Verification items for the finished model (mm, model axes). A direction names the side the tool comes from. Give positions to 0.01 mm unless a question says otherwise; leave off trailing zeros. Loops run counter-clockwise (first coordinate to the right, second up) from the corner with the lowest first, then second, coordinate; pieces in that order, holes last. Notation, with made-up numbers: M -36,15 L 9,15 A23 ccw 9,29 Z; hole C -7.5,7 d7. An arc over 180 degrees is marked long. Use CSV: the item, a comma, the result in double quotes.
from build123d import *

# Parameters (mm, degrees)
SKETCH1_R                   = 20.701
BOSS_EXTRUDE1_DEPTH         = 25.4
SKETCH2_W                   = 25.654
SKETCH2_H                   = 101.6
CUT_EXTRUDE1_DEPTH          = 25.654
F_1_4_20_TAPPED_HOLE1_D     = 5.1054
F_1_4_20_TAPPED_HOLE1_DEPTH = 25.4
F_1_4_20_TAPPED_HOLE1_TIP   = 1.533816902
F_3_8_24_TAPPED_HOLE1_D     = 8.4328
SKETCH10_R                  = 9.525
CUT_EXTRUDE2_DEPTH          = 19.05
CHAMFER1_SIZE               = 1.27


with BuildPart() as part:
    # Sketch1 → Boss-Extrude1 (new, symmetric)
    with BuildSketch(Plane.XY):
        with BuildLine():
            Line((0, 0), (0, 203.2))
            ThreePointArc((0, 203.2), (44.636926547, 310.963073453), (152.4, 355.6))
            Line((152.4, 355.6), (285.75, 355.6))
            Line((285.75, 355.6), (285.75, 254))
            Line((285.75, 254), (203.2, 254))
            ThreePointArc((203.2, 254), (131.357951031, 224.242048969), (101.6, 152.4))
            Line((101.6, 152.4), (101.6, 0))
            Line((101.6, 0), (0, 0))
        make_face()
        with Locations((242.9256, 304.8)):
            Circle(SKETCH1_R, mode=Mode.SUBTRACT)
    extrude(amount=BOSS_EXTRUDE1_DEPTH, both=True)

    # Sketch2 → Cut-Extrude1 (cut)
    with BuildSketch(Plane(origin=(285.75, 0, 0), x_dir=(0, 0, -1), z_dir=(1, 0, 0))):
        with Locations((0, 304.8)):
            Rectangle(SKETCH2_W, SKETCH2_H)
    extrude(amount=-CUT_EXTRUDE1_DEPTH, mode=Mode.SUBTRACT)

    # 1/4-20 Tapped Hole1
    with Locations(Plane(origin=(285.75, 0, 0), x_dir=(0, 0, -1), z_dir=(1, 0, 0))):
        with Locations((19.05, 342.9), (-19.05, 342.9), (-19.05, 266.7), (19.05, 266.7)):
            Hole(F_1_4_20_TAPPED_HOLE1_D / 2, depth=F_1_4_20_TAPPED_HOLE1_DEPTH)
            with Locations((0, 0, -(F_1_4_20_TAPPED_HOLE1_DEPTH + F_1_4_20_TAPPED_HOLE1_TIP / 2))):  # 118° drill point
                Cone(0, F_1_4_20_TAPPED_HOLE1_D / 2, F_1_4_20_TAPPED_HOLE1_TIP, mode=Mode.SUBTRACT)

    # 3/8-24 Tapped Hole1 (through all)
    with Locations(Plane.XY.offset(25.4)):
        with Locations((12.7, 29.21), (12.7, 8.89)):
            Hole(F_3_8_24_TAPPED_HOLE1_D / 2)

    # Sketch10 → Cut-Extrude2 (cut)
    with BuildSketch(Plane(origin=(101.6, 0, 0), x_dir=(0, 0, -1), z_dir=(1, 0, 0))):
        with Locations(Location((0, 19.05, 0), (0, 0, 90))):
            Circle(SKETCH10_R)
    extrude(amount=-CUT_EXTRUDE2_DEPTH, mode=Mode.SUBTRACT)

    # Chamfer1
    chamfer1_edges = [part.edges().sort_by_distance(p)[0] for p in [
        (244.475, 254, -25.4),
        (131.357951031, 224.242048969, -25.4),
        (101.6, 76.2, -25.4),
        (131.357951031, 224.242048969, 25.4),
        (244.475, 254, 25.4),
        (219.075, 355.6, 25.4),
        (44.636926547, 310.963073453, 25.4),
        (0, 101.6, 25.4),
        (0, 101.6, -25.4),
        (101.6, 76.2, 25.4),
        (44.636926547, 310.963073453, -25.4),
        (219.075, 355.6, -25.4),
    ]]
    chamfer(chamfer1_edges, length=CHAMFER1_SIZE)


solid = part.part
(1) Section check A-A on y = 104.5. Record the cut outline in (x, z), plus the area to 3 significant figures.
Calculated:
outline,"M 0,-24.13 L 1.27,-25.4 L 100.33,-25.4 L 101.6,-24.13 L 101.6,24.13 L 100.33,25.4 L 1.27,25.4 L 0,24.13 Z"
area,"5,160 mm²"
(2) Mould release check, pull along Y, two halves, no side actions. Record for faces 4 (the flat face through (236, 254, 0)), 5 (the conical face through (44.2, 309, 25.2)), 6 (the cylindrical face through (13.25, 33.39, -0.36)), 7 (the flat face through (101.6, 77, 0)): released by +Y, released by -Y, zero draft, split by the parting line, or undercut.
Calculated:
face 4,"released by -Y"
face 5,"released by +Y"
face 6,"undercut"
face 7,"zero draft"
(3) Tool access check on faces 1 (the cylindrical face through (92.208, 11.491, -5.796)), 2 (the flat face through (260.096, 336, 0)), 3 (the flat face through (285.75, 306, 19)). Record the directions out of +Z, -Z, +X, -X, +Y, -Y that give a thin tool (end or side, any length) a straight path to the whole face; none if there is none.
Calculated:
face 1,"+X"
face 2,"+X, +Y, -Y"
face 3,"+Z, -Z, +X, +Y, -Y"
(4) Section check B-B on y = 19.05. Record the cut outline in (x, z) (3 decimals).
Calculated:
outline,"M 0,-24.13 L 1.27,-25.4 L 100.33,-25.4 L 101.6,-24.13 L 101.6,-9.525 L 82.55,-9.525 L 82.55,9.525 L 101.6,9.525 L 101.6,24.13 L 100.33,25.4 L 1.27,25.4 L 0,24.13 Z"
(5) Scan lines: L1, parallel to Y at x = 272, z = -19; L2, parallel to Z at x = 278, y = 266.7; L3, parallel to Y at x = 241.5, z = -16. Record each from-to range of solid material in increasing order. Write a range as from..to.
Calculated:
L1,"y = 254..264.15, 269.25..340.35, 345.45..355.6"
L2,"z = -25.4..-21.6, -16.5..-12.83, 12.83..16.5, 21.6..25.4"
L3,"y = 254..284.15, 325.45..355.6"
(6) Depth check by flat-ended pin: pin 1 Ø20.5 at (y, z) = (338, 1.5) entering from +X; pin 2 Ø8 at (y, z) = (285, 2.5) entering from -X; pin 3 Ø4.5 at (y, z) = (342.9, 19.05) entering from -X; pin 4 Ø8 at (y, z) = (342.9, -19.05) entering from +X. Enter the tip coordinate at first touch or a pass-through.
Calculated:
pin 1,"stops at x = 260.1"
pin 2,"stops at x = 21.35"
pin 3,"stops at x = 86.57"
pin 4,"stops at x = 285.75"
